Can you work these out from the model? Positions are in its coordinate system, mm. Face numbers are marked on the shaded views. A direction names the side the tool comes from. Coordinates: 2 decimals unless noted, no trailing zeros. Order: outer loops, then holes, each group sorted by start corner. A loop starts at its lowest first (then second) coordinate and runs counter-clockwise, first axis right, second up. Notation, with made-up numbers: (7, 30.5) -> (66, 30.5) arc R7 ccw to (66, 42.5) -> close; hole circle Ø1 at (-38.5, -1.5). An arc over 180 degrees is marked (long way). Return JSON: item names as keys, results as strings. Group by question number.
1) If we section it at C-C, the plane y = -5.5: Please give me the cut outline in (x, z).
2) If I drill on probe 1 along Y at (x, z) = (-2, 27.5) (3 decimals); probe 2 along Y at (x, z) = (1, 29.05) (3 decimals); probe 3 along Y at (x, z) = (-4.5, 5), over which ranges is the centre line in solid material (lowest first)? Write a range as from..to.
3) If we section it at A-A, the plane y = -12.55: Please give me the cut outline in (x, z) (3 decimals), then the cut area to 3 significant figures.
4) If we section it at B-B, the plane z = 23.5: Please give me the cut outline in (x, y).
5) For the marked faces 1 and 2, which set-ups out of +Z, -Z, +X, -X, +Y, -Y let a thin tool reach every point of the face, with its end or its side?
6) For pin 1 (1 mm diameter, centred on x = -0.5, z = 7.5, fed in from +Y); pin 2 (3 mm diameter, centred on x = -3.5, y = -13, fed in from -Z); pin 3 (2.5 mm diameter, centred on x = 1, y = -12.55, fed in from +Z); pin 4 (4 mm diameter, centred on y = -12, z = 24.5, fed in from -X), each with a flat end and sliding along its axis, tell me the tip position at first contact or that it passes through.
7) If we section it at D-D, the plane x = -2.75: State how many separate pieces and enclosed holes the cut face has, then the cut area to 3 significant figures.
8) Thinking about a two-plate mould opening in X: for the marked faces 3, 4, 5 and 6, which applies, +X half, -X half, draft (parallel to the pull), parting line (faces both ways), or undercut?
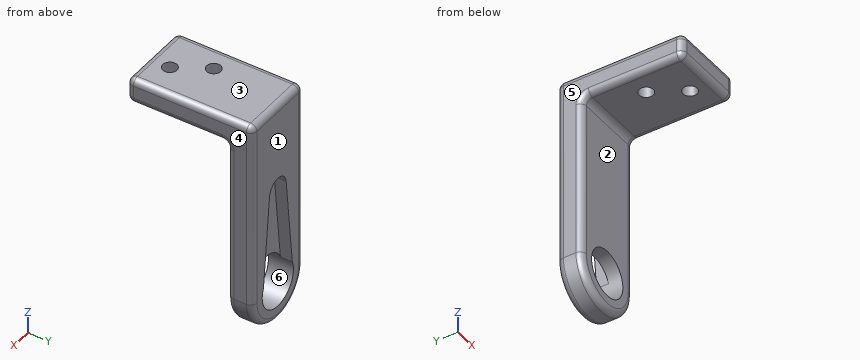
from build123d import *

# Parameters (mm, degrees)
PITCH_ARM_BASE_DEPTH          = 4
PITCH_ARM_MOUNTING_HOLE_REACH = 32.854
SKETCH2_R                     = 3.75
PITCH_ARM_SLOT_DEPTH          = 1.9
SKETCH5_W                     = 12
SKETCH5_H                     = 4
MOUNTING_BRACKET_DEPTH        = 16.05
BRACKET_MOUNTING_HOLES_REACH  = 38.299
SKETCH8_R                     = 1.125
F_1MM_FILLETS_R               = 1


with BuildPart() as part:
    # Sketch1 → Pitch Arm Base (new body)
    with BuildSketch(Plane(origin=(0, 0, 0), x_dir=(1, 0, 0), z_dir=(0, 1, 0))):
        with BuildLine():
            Line((-6, 0), (-6, -30))
            Line((-6, -30), (6, -30))
            Line((6, -30), (6, 0))
            ThreePointArc((6, 0), (0, 6), (-6, 0))
        make_face()
    extrude(amount=PITCH_ARM_BASE_DEPTH)

    # Sketch2 → Pitch Arm Mounting Hole (cut, up to next)
    with BuildSketch(Plane(origin=(0, 4, 0), x_dir=(1, 0, 0), z_dir=(0, 1, 0)), mode=Mode.PRIVATE) as pitch_arm_mounting_hole_sk1:
        with Locations(Location((0, 0, 0), (0, 0, 270))):
            Circle(SKETCH2_R)
    pitch_arm_mounting_hole_tool1 = extrude(pitch_arm_mounting_hole_sk1.sketch, amount=-PITCH_ARM_MOUNTING_HOLE_REACH, mode=Mode.PRIVATE) & part.part
    add(pitch_arm_mounting_hole_tool1.solids().sort_by_distance((0, 4, 0))[0], mode=Mode.SUBTRACT)

    # Sketch4 → Pitch Arm Slot (cut)
    with BuildSketch(Plane(origin=(0, 4, 0), x_dir=(1, 0, 0), z_dir=(0, 1, 0))):
        with BuildLine():
            Line((-3.46, -1.445994467), (-1.989882432, -16.005994467))
            ThreePointArc((-1.989882432, -16.005994467), (0, -17.805076808), (1.989882432, -16.005994467))
            Line((1.989882432, -16.005994467), (3.46, -1.445994467))
            ThreePointArc((3.46, -1.445994467), (0, -3.75), (-3.46, -1.445994467))
        make_face()
    extrude(amount=-PITCH_ARM_SLOT_DEPTH, mode=Mode.SUBTRACT)

    # Sketch5 → Mounting Bracket (add)
    with BuildSketch(Plane.XZ):
        with Locations((0, 28)):
            Rectangle(SKETCH5_W, SKETCH5_H)
    extrude(amount=MOUNTING_BRACKET_DEPTH)

    # Sketch8 → Bracket Mounting Holes (cut, up to next)
    with BuildSketch(Plane(origin=(0, 0, 26), x_dir=(-1, 0, 0), z_dir=(0, 0, -1)), mode=Mode.PRIVATE) as bracket_mounting_holes_sk1:
        with Locations((-1, -12.55)):
            Circle(SKETCH8_R)
    bracket_mounting_holes_tool1 = extrude(bracket_mounting_holes_sk1.sketch, amount=-BRACKET_MOUNTING_HOLES_REACH, mode=Mode.PRIVATE) & part.part
    # Sketch8 → Bracket Mounting Holes (cut, up to next)
    with BuildSketch(Plane(origin=(0, 0, 26), x_dir=(-1, 0, 0), z_dir=(0, 0, -1)), mode=Mode.PRIVATE) as bracket_mounting_holes_sk2:
        with Locations((2, -7.55)):
            Circle(SKETCH8_R)
    bracket_mounting_holes_tool2 = extrude(bracket_mounting_holes_sk2.sketch, amount=-BRACKET_MOUNTING_HOLES_REACH, mode=Mode.PRIVATE) & part.part
    add(bracket_mounting_holes_tool1.solids().sort_by_distance((1, -12.55, 26))[0], mode=Mode.SUBTRACT)
    add(bracket_mounting_holes_tool2.solids().sort_by_distance((-2, -7.55, 26))[0], mode=Mode.SUBTRACT)

    # 1mm Fillets
    f_1mm_fillets_edges = [part.edges().sort_by_distance(p)[0] for p in [
        (0, 4, 30),
        (6, 4, 15),
        (6, 0, 13),
        (0, 0, 26),
        (-6, -8.025, 26),
        (6, -8.025, 26),
        (-6, -16.05, 28),
        (0, -16.05, 26),
        (6, -16.05, 28),
        (0, -16.05, 30),
        (0, 4, -6),
        (-6, 0, 13),
        (0, 0, -6),
        (6, -6.025, 30),
        (-6, -6.025, 30),
        (-6, 4, 15),
    ]]
    fillet(f_1mm_fillets_edges, radius=F_1MM_FILLETS_R)


solid = part.part
Result sheet:
{
 "1": {"outline": "(-6, 27) arc R1 ccw to (-5, 26) -> (5, 26) arc R1 ccw to (6, 27) -> (6, 29) arc R1 ccw to (5, 30) -> (-5, 30) arc R1 ccw to (-6, 29) -> close"},
 "2": {"probe 1": "y = -16.05..-8.675, -6.425..4", "probe 2": "y = -16.049..-13.675, -11.425..3.999", "probe 3": "y = 0..4"},
 "3": {"outline": "(-6, 27) arc R1 ccw to (-5, 26) -> (-0.125, 26) -> (-0.125, 30) -> (-5, 30) arc R1 ccw to (-6, 29) -> close; (2.125, 26) -> (5, 26) arc R1 ccw to (6, 27) -> (6, 29) arc R1 ccw to (5, 30) -> (2.125, 30) -> close", "area": "38.1 mm2"},
 "4": {"outline": "(-6, 1) arc R1 ccw to (-5, 0) -> (5, 0) arc R1 ccw to (6, 1) -> (6, 3) arc R1 ccw to (5, 4) -> (-5, 4) arc R1 ccw to (-6, 3) -> close"},
 "5": {"face 1": "+Z, -Z, +X, -X, +Y", "face 2": "-Z, +X, -X, -Y"},
 "6": {"pin 1": "stops at y = 2.1", "pin 2": "stops at z = 26", "pin 3": "stops at z = 30", "pin 4": "stops at x = -5.87"},
 "7": {"separate pieces": "3", "enclosed holes": "0", "area": "166 mm2"},
 "8": {"face 3": "draft", "face 4": "+X half", "face 5": "-X half", "face 6": "undercut"}
}
